```python
from build123d import *

# Parameters (mm, degrees)
F0_W     = 5.2
F0_H     = 226.71
F1_DEPTH = 2
F3_DEPTH = 4.5
F4_W     = 1.2
F4_H     = 2.1
F5_DEPTH = 25
F6_W     = 183
F6_H     = 227.71
F7_DEPTH = 1
F8_W     = 2
F8_H     = 226.71
F9_DEPTH = 1
F10_SIZE = 1


# Not quite as in the source:
# - a feature names something its author has since deleted; it is built from what else it names


with BuildPart() as f1:
    # F0 (on Top) → F1 (new body)
    with BuildSketch(Plane.XY):
        with Locations((2.6, 113.355)):
            Rectangle(F0_W, F0_H)
    extrude(amount=F1_DEPTH)

    # F2 (on face) → F3 (join)
    with BuildSketch(Plane.XY.offset(2)):
        Polygon((0, 226.71), (0, 0), (2, 0), (2, 224.71), (3.2, 224.71), (3.2, 0), (5.2, 0), (5.2, 226.71), align=None)
    extrude(amount=F3_DEPTH)


with BuildPart() as f1b:
    # F0 (on Top) → F1, piece 2 (new body)
    with BuildSketch(Plane.XY):
        with Locations((63.6, 113.355)):
            Rectangle(F0_W, F0_H)
    extrude(amount=F1_DEPTH)

    # F2 (on face) → F3, piece 2 (join)
    with BuildSketch(Plane.XY.offset(2)):
        Polygon((61, 226.71), (61, 0), (63, 0), (63, 224.71), (64.2, 224.71), (64.2, 0), (66.2, 0), (66.2, 226.71), align=None)
    extrude(amount=F3_DEPTH)


with BuildPart() as f5_tool:
    # F4 (on face) → F5 (new body)
    with BuildSketch(Plane.XY.offset(2)):
        with Locations((2.6, 2.95)):
            Rectangle(F4_W, F4_H)
        with Locations((63.6, 2.95)):
            Rectangle(F4_W, F4_H)
    extrude(amount=-F5_DEPTH)


with BuildPart() as f1_1:
    add(f1.part)

    # F5: cut by f5_tool
    add(f5_tool.part, mode=Mode.SUBTRACT)



with BuildPart() as f1b_1:
    add(f1b.part)

    # F5: cut by f5_tool
    add(f5_tool.part, mode=Mode.SUBTRACT)


with BuildPart() as f1_2:
    add(f1_1.part)

    add(f1b_1.part)  # F7 merges F1b
    # F6 (on Top) → F7 (join)
    with BuildSketch(Plane.XY):
        with Locations((33.2, 113.855)):
            Rectangle(F6_W, F6_H)
    extrude(amount=-F7_DEPTH)

    # F8 (on face) → F9 (join)
    with BuildSketch(Plane.XY):
        with Locations((-53.8, 113.355)):
            Rectangle(F8_W, F8_H)
    extrude(amount=F9_DEPTH)

    # F10
    f10_edges = [f1_2.edges().sort_by_distance(p)[0] for p in [
        (2.6, 0, 2),
        (63.6, 0, 2),
    ]]
    chamfer(f10_edges, length=F10_SIZE)


solid = f1_2.part
```
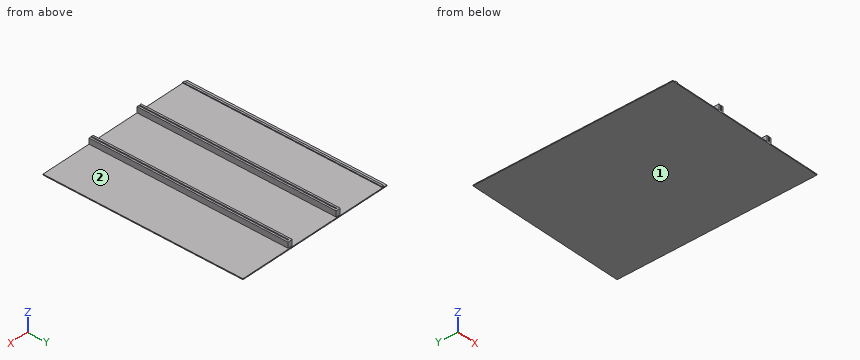
For this review, take the finished solid that the model builds, in its own axes (mm). Face numbers are marked on the shaded views. Coordinates: 2 decimals unless noted, no trailing zeros. Order: outer loops, then holes, each group sorted by start corner. A loop starts at its lowest first (then second) coordinate and runs counter-clockwise, first axis right, second up. Notation, with made-up numbers: (43, 10) - (50, 10) arc R31 ccw to (50, 34) - close; hole circle Ø2 at (56.5, 9). An arc over 180 degrees is marked (long way). Answer as a JSON object with one key per item and string values. Group by question number.
1. We need section B-B on y = 201. State the section outline as (x, z) points, then the cut area to 3 significant figures.
2. The part is to be moulded in two halves that separate along X. For the marked faces 1 and 2, say which applies: pulls with the +X half, pulls with the -X half, needs draft (parallel to the pull), parting line crosses it, or undercut.
3. For probe 1 along X at (y, z) = (160.5, 3.5); probe 2 along X at (y, z) = (57, 0.5); probe 3 along X at (y, z) = (101.5, 1.75), list the stretches that pass through material, from the lowest coordinate up.
4. We need section C-C on x = -25.5. State the section outline as (y, z) points.
5. We need section A-A on z = 4.5. State the section outline as (x, y) points, then the cut area to 3 significant figures.
6. Clearance check with flat-ended pins moving along their axes: P1, Ø0.6, axis at x = 63.5, y = 3.5, coming from the +Z side; P2, Ø1.6, axis at x = -54, y = 75.5, coming from the +Z side; P3, Ø0.5, axis at x = -53.5, z = 0.5, coming from the +Y side. State where each tip first meets the part, or that it passes through.
Final values:
{
 "1": {"outline": "(-58.3, -1) - (124.7, -1) - (124.7, 0) - (66.2, 0) - (66.2, 6.5) - (64.2, 6.5) - (64.2, 2) - (63, 2) - (63, 6.5) - (61, 6.5) - (61, 0) - (5.2, 0) - (5.2, 6.5) - (3.2, 6.5) - (3.2, 2) - (2, 2) - (2, 6.5) - (0, 6.5) - (0, 0) - (-52.8, 0) - (-52.8, 1) - (-54.8, 1) - (-54.8, 0) - (-58.3, 0) - close", "area": "242 mm²"},
 "2": {"face 1": "needs draft", "face 2": "undercut"},
 "3": {"probe 1": "0 to 2, 3.2 to 5.2, 61 to 63, 64.2 to 66.2", "probe 2": "-54.8 to -52.8, 0 to 5.2, 61 to 66.2", "probe 3": "0 to 5.2, 61 to 66.2"},
 "4": {"outline": "(0, -1) - (227.71, -1) - (227.71, 0) - (0, 0) - close"},
 "5": {"outline": "(0, 0) - (2, 0) - (2, 224.71) - (3.2, 224.71) - (3.2, 0) - (5.2, 0) - (5.2, 226.71) - (0, 226.71) - close; (61, 0) - (63, 0) - (63, 224.71) - (64.2, 224.71) - (64.2, 0) - (66.2, 0) - (66.2, 226.71) - (61, 226.71) - close", "area": "1,820 mm²"},
 "6": {"P1": "z = 0", "P2": "z = 1", "P3": "y = 226.71"}
}
